from build123d import *

# Parameters (mm, degrees)
F1_DEPTH = 4
F3_D     = 6.6
F4_R     = 3


with BuildPart() as f1:
    # F0 (on Front) → F1 (new body)
    with BuildSketch(Plane.XZ):
        with BuildLine():
            Line((-33.4687721395, 93.1710324697), (-32.4545669232, 90.3476678494))
            ThreePointArc((-32.4545669232, 90.3476678494), (-32.0483511021, 90.4925587639), (-31.6414884556, 90.6356232853))
            ThreePointArc((-31.6414884556, 90.6356232853), (-28.6634875045, 91.6209827718), (-25.6548841035, 92.508523508))
            Line((-25.6548841035, 92.508523508), (-26.4565992317, 95.3994148677))
            ThreePointArc((-26.4565992318, 95.3994148677), (-29.9833946631, 94.350389742), (-33.4687721395, 93.1710324697))
        make_face()
        with BuildLine():
            ThreePointArc((0, 99), (-13.3502420971, 98.0957238413), (-26.4565992318, 95.3994148677))
            Line((-26.4565992317, 95.3994148677), (-25.6548841035, 92.508523508))
            ThreePointArc((-25.6548841035, 92.508523508), (-22.7517340683, 93.2649912716), (-19.8263642502, 93.9303746432))
            ThreePointArc((-19.8263642502, 93.9303746432), (-13.3908139049, 95.0614859076), (-6.8932268351, 95.7521980103))
            ThreePointArc((-6.8932268351, 95.7521980103), (-3.4488397334, 95.9380295008), (0, 96))
            Line((0, 96), (0, 99))
        make_face()
        with BuildLine():
            ThreePointArc((-19.8263642502, 93.9303746432), (-22.7517340683, 93.2649912716), (-25.6548841035, 92.508523508))
            Line((-25.6548841035, 92.508523508), (-23.5169770949, 84.7994798824))
            ThreePointArc((-23.5169770949, 84.7994798824), (-20.6124161637, 85.5519041278), (-17.6838927225, 86.2048718935))
            Line((-17.6838927225, 86.2048718935), (-19.8263642502, 93.9303746432))
        make_face()
        with BuildLine():
            ThreePointArc((-25.6548841035, 92.508523508), (-28.6634875045, 91.6209827718), (-31.6414884556, 90.6356232853))
            Line((-31.6414884556, 90.6356232853), (-29.240736677, 82.9998754131))
            ThreePointArc((-29.240736677, 82.9998754131), (-26.3941988829, 83.9484738714), (-23.5169770949, 84.7994798824))
            Line((-23.5169770949, 84.7994798824), (-25.6548841035, 92.508523508))
        make_face()
        with BuildLine():
            ThreePointArc((-23.5169770949, 84.7994798824), (-26.3941988829, 83.9484738714), (-29.240736677, 82.9998754131))
            ThreePointArc((-29.240736677, 82.9998754131), (-26.3820624935, 79.5277358011), (-21.9135468384, 79.0176971631))
            Line((-21.9135468384, 79.0176971631), (-23.5169770949, 84.7994798824))
        make_face()
        with BuildLine():
            Line((-23.5169770949, 84.7994798824), (-21.9135468384, 79.0176971631))
            ThreePointArc((-21.9135468384, 79.0176971631), (-18.3459706544, 81.7563413064), (-17.6838927225, 86.2048718935))
            ThreePointArc((-17.6838927225, 86.2048718935), (-20.6124161637, 85.5519041278), (-23.5169770949, 84.7994798824))
        make_face()
        with BuildLine():
            Line((0, 88), (0, 96))
            ThreePointArc((0, 96), (-3.4488397334, 95.9380295008), (-6.8932268351, 95.7521980103))
            Line((-6.8932268351, 95.7521980103), (-5.9965124161, 87.7954545455))
            ThreePointArc((-5.9965124161, 87.7954545455), (-3, 87.9488487702), (0, 88))
        make_face()
        with BuildLine():
            ThreePointArc((6.2693850791, 95.7950667348), (3.1363668039, 95.9487530053), (0, 96))
            Line((0, 96), (0, 88))
            ThreePointArc((0, 88), (3, 87.9488487702), (5.9965124161, 87.7954545455))
            Line((5.9965124161, 87.7954545455), (6.2693850791, 95.7950667348))
        make_face()
        with BuildLine():
            Line((0, 88), (0, 82))
            ThreePointArc((0, 82), (4.1696958686, 83.685647631), (5.9965124161, 87.7954545455))
            ThreePointArc((5.9965124161, 87.7954545455), (3, 87.9488487702), (0, 88))
        make_face()
        with BuildLine():
            ThreePointArc((-5.9965124161, 87.7954545455), (-4.1696958686, 83.685647631), (0, 82))
            Line((0, 82), (0, 88))
            ThreePointArc((0, 88), (-3, 87.9488487702), (-5.9965124161, 87.7954545455))
        make_face()
        with BuildLine():
            ThreePointArc((26.4565992318, 95.3994148677), (13.3502420971, 98.0957238413), (0, 99))
            Line((0, 99), (0, 96))
            ThreePointArc((0, 96), (3.1363668039, 95.9487530053), (6.2693850791, 95.7950667348))
            ThreePointArc((6.2693850791, 95.7950667348), (12.9456893063, 95.1231261491), (19.5587476854, 93.9864638604))
            ThreePointArc((19.5587476854, 93.9864638604), (22.6188903752, 93.2972979147), (25.6548841035, 92.508523508))
            Line((25.6548841035, 92.508523508), (26.4565992317, 95.3994148677))
        make_face()
        with BuildLine():
            Line((-35.4971825722, 98.8177617103), (-36.5113877886, 101.6411263306))
            ThreePointArc((-36.5113877886, 101.6411263306), (-40.1297065965, 93.9659866573), (-32.4545669232, 90.3476678494))
            Line((-32.4545669232, 90.3476678494), (-33.4687721395, 93.1710324697))
            ThreePointArc((-33.4687721395, 93.1710324697), (-37.3063419762, 94.9801918737), (-35.4971825722, 98.8177617103))
        make_face()
        with BuildLine():
            ThreePointArc((-28.8617446165, 104.0720889465), (-32.7091578143, 102.9276979004), (-36.5113877886, 101.6411263306))
            Line((-36.5113877886, 101.6411263306), (-35.4971825722, 98.8177617103))
            ThreePointArc((-35.4971825722, 98.8177617103), (-31.8005700973, 100.068595181), (-28.0600294882, 101.1811975869))
            Line((-28.0600294882, 101.1811975869), (-28.8617446165, 104.0720889465))
        make_face()
        with BuildLine():
            ThreePointArc((0, 108), (-14.5639004696, 107.0135169178), (-28.8617446165, 104.0720889465))
            Line((-28.8617446165, 104.0720889465), (-28.0600294882, 101.1811975869))
            ThreePointArc((-28.0600294882, 101.1811975869), (-14.1593476787, 104.0409192256), (0, 105))
            Line((0, 105), (0, 108))
        make_face()
        with BuildLine():
            ThreePointArc((28.8617446165, 104.0720889465), (14.5639004696, 107.0135169178), (0, 108))
            Line((0, 108), (0, 105))
            ThreePointArc((0, 105), (14.1593476787, 104.0409192256), (28.0600294882, 101.1811975869))
            Line((28.0600294882, 101.1811975869), (28.8617446165, 104.0720889465))
        make_face()
        with BuildLine():
            ThreePointArc((37.3643109139, 101.3306877009), (33.1413854263, 102.789340751), (28.8617446165, 104.0720889465))
            Line((28.8617446165, 104.0720889465), (28.0600294882, 101.1811975869))
            ThreePointArc((28.0600294882, 101.1811975869), (32.2207913867, 99.9340812857), (36.3264133885, 98.5159463758))
            Line((36.3264133885, 98.5159463758), (37.3643109139, 101.3306877009))
        make_face()
        with BuildLine():
            ThreePointArc((33.2127208123, 90.0717224008), (40.9179985132, 93.62541), (37.3643109139, 101.3306877009))
            Line((37.3643109139, 101.3306877009), (36.3264133885, 98.5159463758))
            ThreePointArc((36.3264133885, 98.5159463758), (38.1032571881, 94.6633075254), (34.2506183377, 92.8864637258))
            Line((34.2506183377, 92.8864637258), (33.2127208123, 90.0717224008))
        make_face()
        with BuildLine():
            ThreePointArc((32.2010471833, 90.4383356785), (32.7073976674, 90.2564465167), (33.2127208123, 90.0717224008))
            Line((33.2127208123, 90.0717224008), (34.2506183377, 92.8864637258))
            ThreePointArc((34.2506183377, 92.8864637258), (30.3796033074, 94.2235623551), (26.4565992318, 95.3994148677))
            Line((26.4565992317, 95.3994148677), (25.6548841035, 92.508523508))
            ThreePointArc((25.6548841035, 92.508523508), (28.9464784677, 91.5319691928), (32.2010471833, 90.4383356785))
        make_face()
        with BuildLine():
            ThreePointArc((23.5169770949, 84.7994798824), (26.3941988829, 83.9484738714), (29.240736677, 82.9998754131))
            Line((29.240736677, 82.9998754131), (32.2010471833, 90.4383356785))
            ThreePointArc((32.2010471833, 90.4383356785), (28.9464784677, 91.5319691928), (25.6548841035, 92.508523508))
            Line((25.6548841035, 92.508523508), (23.5169770949, 84.7994798824))
        make_face()
        with BuildLine():
            ThreePointArc((17.6838927225, 86.2048718935), (20.6124161637, 85.5519041278), (23.5169770949, 84.7994798824))
            Line((23.5169770949, 84.7994798824), (25.6548841035, 92.508523508))
            ThreePointArc((25.6548841035, 92.508523508), (22.6188903752, 93.2972979147), (19.5587476854, 93.9864638604))
            Line((19.5587476854, 93.9864638604), (17.6838927225, 86.2048718935))
        make_face()
        with BuildLine():
            ThreePointArc((17.6838927225, 86.2048718935), (18.3459706544, 81.7563413064), (21.9135468384, 79.0176971631))
            Line((21.9135468384, 79.0176971631), (23.5169770949, 84.7994798824))
            ThreePointArc((23.5169770949, 84.7994798824), (20.6124161637, 85.5519041278), (17.6838927225, 86.2048718935))
        make_face()
        with BuildLine():
            Line((23.5169770949, 84.7994798824), (21.9135468384, 79.0176971631))
            ThreePointArc((21.9135468384, 79.0176971631), (26.3820624935, 79.5277358011), (29.240736677, 82.9998754131))
            ThreePointArc((29.240736677, 82.9998754131), (26.3941988829, 83.9484738714), (23.5169770949, 84.7994798824))
        make_face()
    extrude(amount=F1_DEPTH)

    # F3 (through all)
    with Locations(Plane.XZ.offset(4)):
        with Locations((-23.5169770949, 84.7994798824), (0, 87.7954545455), (23.5169770949, 84.7994798824)):
            Hole(F3_D / 2)

    # F4
    f4_edges = [f1.edges().sort_by_distance(p)[0] for p in [
        (-19.826364, -2, 93.930375),
        (6.269385, -2, 95.795067),
        (-31.641488, -2, 90.635623),
        (-6.893227, -2, 95.752198),
        (19.558748, -2, 93.986464),
        (32.201047, -2, 90.438336),
    ]]
    fillet(f4_edges, radius=F4_R)


solid = f1.part
Geometry: final body of the model. Coordinates: model frame, mm. A direction names the side the tool comes from. Coordinates: 2 decimals unless noted, no trailing zeros. Order: outer loops, then holes, each group sorted by start corner. A loop starts at its lowest first (then second) coordinate and runs counter-clockwise, first axis right, second up. Notation, with made-up numbers: M 32,79.25 L 85,79.25 A25 ccw 85,105.25 Z; hole C 63,48 d11. An arc over 180 degrees is marked long. One line per question, with ' | ' between items. Start each with the question number.
Item 1: Cut plane B-B, the plane x = 30. Return the cut outline in (y, z).
Item 2: Draft query along Z for faces 4 (the cylindrical face through (38.125, -1.972, 94.725)), 5 (the cylindrical face through (-13.276, -1.972, 95.078)), 6 (the flat face through (0, 0, 94)). Return one class per face: released by +Z, released by -Z, zero draft, split by the parting line, or undercut.
Item 3: Pin query (flat end, axial travel): pin 1 Ø8.5 at (x, z) = (-23.52, 84.8) entering from +Y; pin 2 Ø6 at (x, z) = (23.52, 84.8) entering from +Y. Return the tip coordinate at first contact, or that it passes through.
Item 4: Cut plane C-C, the plane x = 2. Return the cut outline in (y, z), then the cut area to 3 significant figures.
Item 5: Cut plane A-A, the plane z = 97.25. Return the cut outline in (x, y), then the cut area to 3 significant figures.
Item 6: Set-up query: faces 1 (the flat face through (0, -4, 94)), 2 (the flat face through (18.26, -1.97, 88.6)), 3 (the cylindrical face through (12.9, -1.97, 95.13)). Return all of +Z, -Z, +X, -X, +Y, -Y with unobstructed straight access to the full face (end or side cutting, diameter ignored); none if empty.
Item 7: Ray query, probe 1 along X at (y, z) = (-2.4, 90.75); probe 2 along X at (y, z) = (-2, 92); probe 3 along X at (y, z) = (-1, 85.75). Return the intervals inside material, ascending. Write a range as [from, to].
Item 8: Cut plane D-D, the plane y = -3. Count the separate pieces of the cut face and the enclosed holes in it, then the cut area to 3 significant figures.
A:
1) outline: M -4,84.91 L 0,84.91 L 0,94.35 L -4,94.35 Z; M -4,100.62 L 0,100.62 L 0,103.75 L -4,103.75 Z
2) face 4: undercut | face 5: released by -Z | face 6: zero draft
3) pin 1: stops at y = 0 | pin 2: passes through
4) outline: M -4,82.34 L 0,82.34 L 0,85.17 L -4,85.17 Z; M -4,90.42 L 0,90.42 L 0,98.98 L -4,98.98 Z; M -4,104.98 L 0,104.98 L 0,107.98 L -4,107.98 Z | area: 57.5 mm2
5) outline: M -40.35,-4 L -37.21,-4 L -37.21,0 L -40.35,0 Z; M -18.53,-4 L 18.53,-4 L 18.53,0 L -18.53,0 Z; M 37.86,-4 L 41.09,-4 L 41.09,0 L 37.86,0 Z | area: 174 mm2
6) face 1: +Z, -Z, +X, -X, -Y | face 2: +Y, -Y | face 3: -Z, +Y, -Y
7) probe 1: x = [-37.4, -18.94], [-6.33, -1.47], [1.47, 6.1], [18.78, 38.68] | probe 2: x = [-38.96, -19.04], [-6.47, 6.14], [18.88, 40.01] | probe 3: x = [-30.11, -26.68], [-20.36, -17.59], [-5.56, -2.59], [2.59, 5.56], [17.59, 20.36], [26.68, 30.34]
8) separate pieces: 1 | enclosed holes: 4 | area: 887 mm2
